Answer from the drawing. Dimensions are ordinates in mm from the lowest x, y and z of the part. A direction names the side the tool comes from. Give positions to 0.01 mm unless a question says otherwise; leave off trailing zeros. Loops run counter-clockwise (first coordinate to the right, second up) from the corner with the lowest first, then second, coordinate; pieces in that order, holes last. Notation, with made-up numbers: (75.25, -4.75) - (119.25, -4.75) arc R32 ccw to (119.25, 22.25) - close; hole circle Ø8 at (53, 84.5). An arc over 180 degrees is marked (long way). Write each question's results on one line, items separated by ' | '. Start each with the question number.
Q1. The part is cut by section A-A, the plane y = 6. Write down the section's boundary in (x, z).
Q2. Determine the mould class of the marked faces 4, 5, 6 and 7 for opening direction X: +X half, -X half, draft (parallel to the pull), parting line (faces both ways), or undercut.
Q3. Given pin 1 (3.5 mm diameter, centred on x = 5.5, y = 7.5, fed in from +Z); pin 2 (3.5 mm diameter, centred on y = 6.5, z = 3.5, fed in from -X); pin 3 (1.5 mm diameter, centred on y = 2.5, z = 4, fed in from -X), each flat-ended and moving along its own axis, determine where each tip first touches the part or whether it passes through.
Q4. The part is cut by section D-D, the plane y = 11.25. Write down the section's boundary in (x, z).
Q5. The part is cut by section B-B, the plane x = 6. Write down the section's boundary in (y, z).
Q6. Find the intervals of material crossed by line 1 (X direction, y = 6, z = 2.45); line 2 (X direction, y = 6, z = 1.4); line 3 (Y direction, x = 7.25, z = 5), in increasing order. Write a range as from..to.
Q7. The part is cut by section C-C, the plane z = 0.5. Write down the section's boundary in (x, y).
Q8. For the marked faces 1, 2 and 3, determine the directions among +Z, -Z, +X, -X, +Y, -Y from which every point of the face is accessible in a straight line to the end or side of a thin tool.
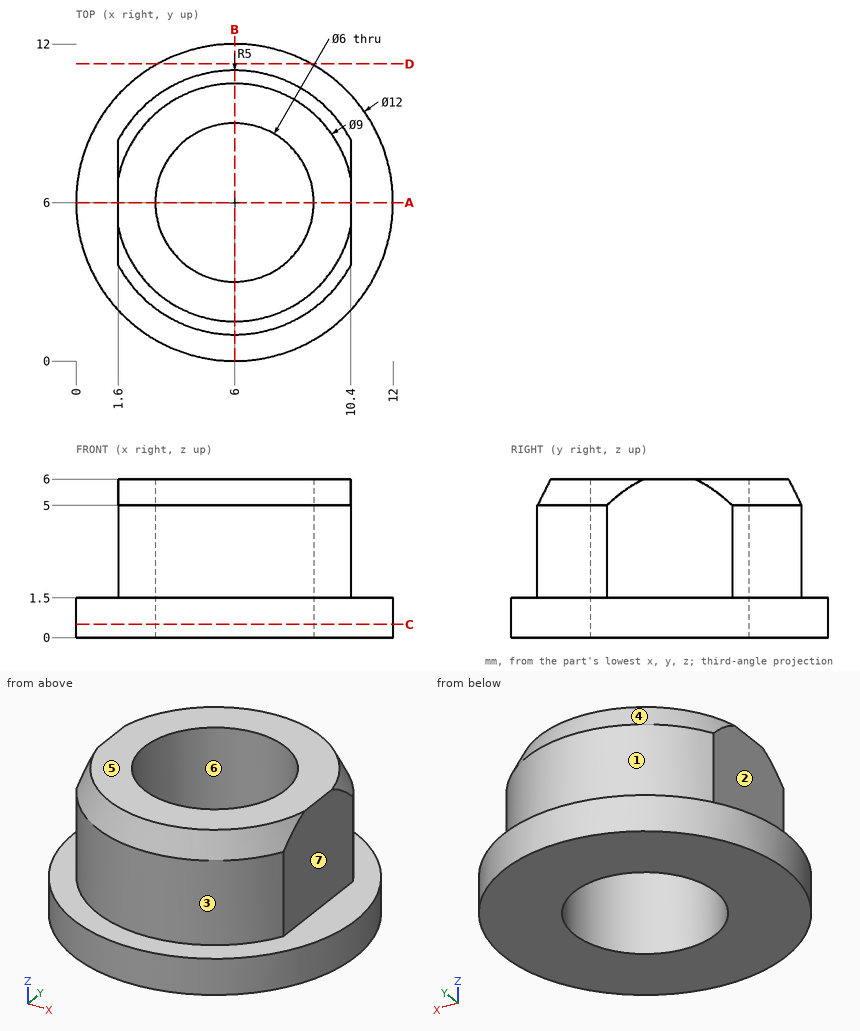
Check sheet entries:
1) outline: (0, 0) - (3, 0) - (3, 6) - (1.6, 6) - (1.6, 1.5) - (0, 1.5) - close; (9, 0) - (12, 0) - (12, 1.5) - (10.4, 1.5) - (10.4, 6) - (9, 6) - close
2) face 4: parting line | face 5: draft | face 6: undercut | face 7: +X half
3) pin 1: stops at z = 6 | pin 2: stops at x = 1.6 | pin 3: stops at x = 1.82
4) outline: (3.1, 0) - (8.9, 0) - (8.9, 1.5) - (3.1, 1.5) - close
5) outline: (0, 0) - (3, 0) - (3, 6) - (1.5, 6) - (1, 5) - (1, 1.5) - (0, 1.5) - close; (9, 0) - (12, 0) - (12, 1.5) - (11, 1.5) - (11, 5) - (10.5, 6) - (9, 6) - close
6) line 1: x = 1.6..3, 9..10.4 | line 2: x = 0..3, 9..12 | line 3: y = 1.16..3.27, 8.73..10.84
7) outline: circle Ø12 at (6, 6); hole circle Ø6 at (6, 6)
8) face 1: +Z, +Y | face 2: +Z, -X, +Y, -Y | face 3: +Z, -Y
